Model file for the job. Use its own axes, mm. A direction names the side the tool comes from. Give positions to 0.01 mm unless a question says otherwise; leave off trailing zeros. Loops run counter-clockwise (first coordinate to the right, second up) from the corner with the lowest first, then second, coordinate; pieces in that order, holes last. Notation, with made-up numbers: (85.5, 3.5) -> (124.5, 3.5) arc R25 cw to (124.5, 21.5) -> close; hole circle Ø1 at (-38.5, 21). An arc over 180 degrees is marked (long way). Use CSV: the item, a comma, the result in double quotes. Start each with the question number.
(1) Cut at B-B on z = 12.5. Write the cut outline in (x, y) (3 decimals), then the cut area to 3 significant figures.
(2) Flat gauge pins, fed straight in: pin 1 (7.5 mm diameter, centred on x = -45, y = 28.5, fed in from -Z); pin 2 (10 mm diameter, centred on y = 6, z = 6.5, fed in from +X); pin 3 (9.5 mm diameter, centred on x = 10, z = 24, fed in from +Y); pin 4 (12 mm diameter, centred on y = 6.5, z = 25.5, fed in from -X). Where does each tip first touch, or does it go through?
(3) 3-axis set-ups, long thin cutter, end or side, ignore diameter. For faces 1 (the flat face through (-38.83, 19.91, 5.02)), 2 (the flat face through (9, 0, 17)), 3 (the cylindrical face through (11.27, -2.58, 2.05)), 4 (the flat face through (-61.576, 33.047, 17.342)): which of +Z, -Z, +X, -X, +Y, -Y reach the whole face in a straight line?
(4) Cut at D-D on x = -50.5. Write the cut outline in (y, z).
(5) Drill centre lines: probe 1 along Z at (x, y) = (12.7, -3.1); probe 2 along Z at (x, y) = (12, -3); probe 3 along Y at (x, z) = (15, 26). Where is each one in solid material? Low to high.
(6) Pull direction Y, two halves, no side cores. Call faces 5 (the cylindrical face through (-61.2, 32.8, 33.4)), 6 (the flat face through (-37.76, 19.3, 17.66)), 7 (the flat face through (9, -5.08, 17)): pulls with the +Y half, pulls with the -Y half, needs draft (parallel to the pull), parting line crosses it, or undercut.
(7) Cut at A-A on x = 12.7. Write the cut outline in (y, z), then the cut area to 3 significant figures.
(8) Cut at C-C on y = 24.5. Write the cut outline in (x, z), then the cut area to 3 significant figures.
from build123d import *

# Parameters (mm, degrees)
SKETCH2_W                       = 19.05
SKETCH2_H                       = 5.08
BOSS_EXTRUDE1_DEPTH             = 35
SKETCH3_W                       = 25
SKETCH3_H                       = 25
CUT_EXTRUDE1_DEPTH              = 38.152489822
F_3_0MM_DOWEL_HOLE1_D           = 3
F_3_0MM_DOWEL_HOLE1_ON_FACE_2_D = 3
F_3_0MM_DOWEL_HOLE1_ON_FACE_3_D = 3
F_3_0MM_DOWEL_HOLE2_D           = 3


with BuildPart() as part:
    # Sketch2 → Boss-Extrude1 (new body)
    with BuildSketch(Plane.XY):
        Polygon((-65.506161542, 32.74), (-63.306457017, 36.55), (-32.995567884, 19.05), (-35.19527241, 15.24), align=None)
        Polygon((-32.995567884, 19.05), (0, 0), (0, -5.08), (-35.19527241, 15.24), align=None)
        with Locations((9.525, -2.54)):
            Rectangle(SKETCH2_W, SKETCH2_H)
    extrude(amount=BOSS_EXTRUDE1_DEPTH)

    # Sketch3 → Cut-Extrude1 (cut, through all)
    with BuildSketch(Plane(origin=(0, 0, 0), x_dir=(0.866025404, -0.5, 0), z_dir=(0.5, 0.866025404, 0))):
        with Locations((-56.1, -17.5)):
            Rectangle(SKETCH3_W, SKETCH3_H)
        Polygon((-67.35, -3.75), (-68.6, -5), (-43.6, -5), (-44.85, -3.75), align=None)
        Polygon((-68.6, -30), (-68.6, -5), (-69.85, -6.25), (-69.85, -28.75), align=None)
        Polygon((-42.35, -6.25), (-43.6, -5), (-43.6, -30), (-42.35, -28.75), align=None)
        Polygon((-43.6, -30), (-68.6, -30), (-67.35, -31.25), (-44.85, -31.25), align=None)
    extrude(amount=-CUT_EXTRUDE1_DEPTH, mode=Mode.SUBTRACT)

    # Ø3.0mm Dowel Hole1 (through all)
    with Locations(Plane(origin=(-61.141393507, 35.3, 2.5), x_dir=(0.866025404, -0.5, 0), z_dir=(0.5, 0.866025404, 0))):
        with Locations((0, 0)):
            Hole(F_3_0MM_DOWEL_HOLE1_D / 2)

    # Ø3.0mm Dowel Hole1 on face 2 (through all)
    with Locations(Plane(origin=(-36.026656797, 20.8, 2.5), x_dir=(0.866025303, -0.500000175, 0), z_dir=(0.500000175, 0.866025303, 0))):
        with Locations((0, 0), (0, -30)):
            Hole(F_3_0MM_DOWEL_HOLE1_ON_FACE_2_D / 2)

    # Ø3.0mm Dowel Hole1 on face 3 (through all)
    with Locations(Plane(origin=(-61.141393507, 35.3, 32.5), x_dir=(0.866025303, -0.500000175, 0), z_dir=(0.500000175, 0.866025303, 0))):
        with Locations((0, 0)):
            Hole(F_3_0MM_DOWEL_HOLE1_ON_FACE_3_D / 2)

    # Ø3.0mm Dowel Hole2 (through all)
    with Locations(Plane(origin=(12.7, 0, 2.5), x_dir=(1, 0, 0), z_dir=(0, 1, 0))):
        with Locations((0, 0), (0, -30)):
            Hole(F_3_0MM_DOWEL_HOLE2_D / 2)


solid = part.part
Check result:
1,outline,"(-65.506, 32.74) -> (-62.692, 31.115) -> (-60.492, 34.925) -> (-63.306, 36.55) -> close; (-38.876, 17.365) -> (0, -5.08) -> (19.05, -5.08) -> (19.05, 0) -> (0, 0) -> (-36.676, 21.175) -> close"
1,area,"303 mm²"
2,pin 1,"z = 0"
2,pin 2,"x = -1.73"
2,pin 3,"y = 0"
2,pin 4,"x = -30.45"
3,face 1,"-X, +Y"
3,face 2,"+Z, -Z, +X, +Y"
3,face 3,"+Y, -Y"
3,face 4,"+X, -Y"
4,outline,"(24.08, 0) -> (29.16, 0) -> (29.16, 3.75) -> (24.08, 3.75) -> close; (24.08, 31.25) -> (29.16, 31.25) -> (29.16, 35) -> (24.08, 35) -> close"
5,probe 1,"0 to 1, 4 to 31, 34 to 35"
5,probe 2,"0 to 1.17, 3.83 to 31.17, 33.83 to 35"
5,probe 3,"-5.08 to 0"
6,face 5,"undercut"
6,face 6,"pulls with the +Y half"
6,face 7,"pulls with the -Y half"
7,outline,"(-5.08, 0) -> (0, 0) -> (0, 1) -> (-5.08, 1) -> close; (-5.08, 4) -> (0, 4) -> (0, 31) -> (-5.08, 31) -> close; (-5.08, 34) -> (0, 34) -> (0, 35) -> (-5.08, 35) -> close"
7,area,"147 mm²"
8,outline,"(-51.23, 0) -> (-42.44, 0) -> (-42.44, 3.75) -> (-51.23, 3.75) -> close; (-51.23, 31.25) -> (-42.44, 31.25) -> (-42.44, 35) -> (-51.23, 35) -> close"
8,area,"66.0 mm²"
